Here's how the part is built. I have some questions about the finished solid (model axes, mm). Face numbers are marked on the shaded views. A direction names the side the tool comes from. Round coordinates to 2 decimals unless told otherwise and drop trailing zeros. Order: outer loops, then holes, each group sorted by start corner. A loop starts at its lowest first (then second) coordinate and runs counter-clockwise, first axis right, second up. Notation, with made-up numbers: (51, 46.5) -> (109, 46.5) arc R27 cw to (109, 76.5) -> close; hole circle Ø5 at (87, 38.5). An arc over 180 degrees is marked (long way). Answer in a Markdown table with one row per item.
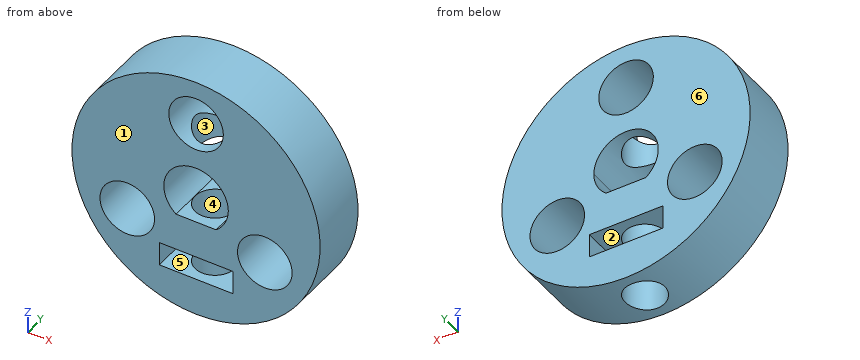
```python
from build123d import *

# Parameters (mm, degrees)
SKETCH1_R                      = 12.5
BOSS_EXTRUDE1_DEPTH            = 6
CUT_EXTRUDE1_REACH             = 20.668
CUT_EXTRUDE2_REACH             = 20.668
SKETCH3_R                      = 2.75
CUT_EXTRUDE3_REACH             = 22.463
SKETCH4_R                      = 2
CUT_EXTRUDE3_DIRECTION_2_REACH = 22.463
CUT_EXTRUDE4_REACH             = 20.668
SKETCH5_W                      = 7.4
SKETCH5_H                      = 2.4


with BuildPart() as part:
    # Sketch1 → Boss-Extrude1 (new body)
    with BuildSketch(Plane(origin=(0, 0, 0), x_dir=(1, 0, 0), z_dir=(0, 1, 0))):
        with Locations(Location((0, 0, 0), (0, 0, 270))):
            Circle(SKETCH1_R)
    extrude(amount=BOSS_EXTRUDE1_DEPTH)

    # Sketch2 → Cut-Extrude1 (cut, up to next)
    with BuildSketch(Plane(origin=(0, 6, 0), x_dir=(1, 0, 0), z_dir=(0, 1, 0)), mode=Mode.PRIVATE) as cut_extrude1_sk1:
        with BuildLine():
            Line((2.014944168, 2.55), (-2.014944168, 2.55))
            ThreePointArc((-2.014944168, 2.55), (-1.416674178, -2.924984491), (3.25, 0))
            ThreePointArc((3.25, 0), (2.924984491, 1.416674178), (2.014944168, 2.55))
        make_face()
    cut_extrude1_tool1 = extrude(cut_extrude1_sk1.sketch, amount=-CUT_EXTRUDE1_REACH, mode=Mode.PRIVATE) & part.part
    add(cut_extrude1_tool1.solids().sort_by_distance((0, 6, 0.174477))[0], mode=Mode.SUBTRACT)

    # Sketch3 → Cut-Extrude2 (cut, up to next)
    with BuildSketch(Plane(origin=(0, 6, 0), x_dir=(1, 0, 0), z_dir=(0, 1, 0)), mode=Mode.PRIVATE) as cut_extrude2_sk1:
        with Locations(Location((0, -8, 0), (0, 0, 270))):
            Circle(SKETCH3_R)
    cut_extrude2_tool1 = extrude(cut_extrude2_sk1.sketch, amount=-CUT_EXTRUDE2_REACH, mode=Mode.PRIVATE) & part.part
    # Sketch3 → Cut-Extrude2 (cut, up to next)
    with BuildSketch(Plane(origin=(0, 6, 0), x_dir=(1, 0, 0), z_dir=(0, 1, 0)), mode=Mode.PRIVATE) as cut_extrude2_sk2:
        with Locations(Location((-6.92820323, 4, 0), (0, 0, 270))):
            Circle(SKETCH3_R)
    cut_extrude2_tool2 = extrude(cut_extrude2_sk2.sketch, amount=-CUT_EXTRUDE2_REACH, mode=Mode.PRIVATE) & part.part
    # Sketch3 → Cut-Extrude2 (cut, up to next)
    with BuildSketch(Plane(origin=(0, 6, 0), x_dir=(1, 0, 0), z_dir=(0, 1, 0)), mode=Mode.PRIVATE) as cut_extrude2_sk3:
        with Locations(Location((6.92820323, 4, 0), (0, 0, 270))):
            Circle(SKETCH3_R)
    cut_extrude2_tool3 = extrude(cut_extrude2_sk3.sketch, amount=-CUT_EXTRUDE2_REACH, mode=Mode.PRIVATE) & part.part
    add(cut_extrude2_tool1.solids().sort_by_distance((0, 6, 8))[0], mode=Mode.SUBTRACT)
    add(cut_extrude2_tool2.solids().sort_by_distance((-6.928203, 6, -4))[0], mode=Mode.SUBTRACT)
    add(cut_extrude2_tool3.solids().sort_by_distance((6.928203, 6, -4))[0], mode=Mode.SUBTRACT)

    # Sketch4 → Cut-Extrude3 (cut, up to next)
    with BuildSketch(Plane.XY.offset(-2.55), mode=Mode.PRIVATE) as cut_extrude3_sk1:
        with Locations(Location((0, 3, 0), (0, 0, 180))):
            Circle(SKETCH4_R)
    cut_extrude3_tool1 = extrude(cut_extrude3_sk1.sketch, amount=-CUT_EXTRUDE3_REACH, mode=Mode.PRIVATE) & part.part
    add(cut_extrude3_tool1.solids().sort_by_distance((0, 3, -2.55))[0], mode=Mode.SUBTRACT)

    # Sketch4 → Cut-Extrude3 direction 2 (cut, up to next)
    with BuildSketch(Plane.XY.offset(-2.55), mode=Mode.PRIVATE) as cut_extrude3_direction_2_sk1:
        with Locations(Location((0, 3, 0), (0, 0, 180))):
            Circle(SKETCH4_R)
    cut_extrude3_direction_2_tool1 = extrude(cut_extrude3_direction_2_sk1.sketch, amount=CUT_EXTRUDE3_DIRECTION_2_REACH, mode=Mode.PRIVATE) & part.part
    add(cut_extrude3_direction_2_tool1.solids().sort_by_distance((0, 3, -2.55))[0], mode=Mode.SUBTRACT)

    # Sketch5 → Cut-Extrude4 (cut, up to next)
    with BuildSketch(Plane(origin=(0, 6, 0), x_dir=(1, 0, 0), z_dir=(0, 1, 0)), mode=Mode.PRIVATE) as cut_extrude4_sk1:
        with Locations((0, 7.525)):
            Rectangle(SKETCH5_W, SKETCH5_H)
    cut_extrude4_tool1 = extrude(cut_extrude4_sk1.sketch, amount=-CUT_EXTRUDE4_REACH, mode=Mode.PRIVATE) & part.part
    add(cut_extrude4_tool1.solids().sort_by_distance((0, 6, -7.525))[0], mode=Mode.SUBTRACT)


solid = part.part
```
1. Suppose I cut it at A-A on z = -4. Write out the boundary of the cut face in (x, y), then the cut area to 3 significant figures.
Numbers:
| item | result |
|---|---|
| outline | (-11.84, 0) -> (-9.68, 0) -> (-9.68, 6) -> (-11.84, 6) -> close; (-4.18, 0) -> (4.18, 0) -> (4.18, 6) -> (-4.18, 6) -> close; (9.68, 0) -> (11.84, 0) -> (11.84, 6) -> (9.68, 6) -> close; hole circle Ø4 at (0, 3) |
| area | 63.5 mm2 |
2. For the marked faces 4, 5 and 6, which set-ups out of +Z, -Z, +X, -X, +Y, -Y let a thin tool reach every point of the face, with its end or its side?
Numbers:
| item | result |
|---|---|
| face 4 | -Z |
| face 5 | +Y, -Y |
| face 6 | +Z, -Z, +X, -X, +Y |
3. Suppose I cut it at C-C on y = 4.25. Write out the boundary of the cut face in (x, z) (3 decimals), then the cut area to 3 significant figures.
Numbers:
| item | result |
|---|---|
| outline | (-3.7, -8.725) -> (-3.7, -6.325) -> (-1.561, -6.325) -> (-1.561, -2.55) -> (-2.015, -2.55) arc R3.25 cw to (-1.561, 2.85) -> (-1.561, 5.736) arc R2.75 cw (long way) to (1.561, 5.736) -> (1.561, 2.85) arc R3.25 cw to (2.015, -2.55) -> (1.561, -2.55) -> (1.561, -6.325) -> (3.7, -6.325) -> (3.7, -8.725) -> (1.561, -8.725) -> (1.561, -12.402) arc R12.5 ccw (long way) to (-1.561, -12.402) -> (-1.561, -8.725) -> close; hole circle Ø5.5 at (-6.928, -4); hole circle Ø5.5 at (6.928, -4) |
| area | 340 mm2 |
4. Suppose I cut it at B-B on x = 0. Write out the boundary of the cut face in (y, z) (3 decimals), then the cut area to 3 significant figures.
Numbers:
| item | result |
|---|---|
| outline | (0, -12.5) -> (1, -12.5) -> (1, -8.725) -> (0, -8.725) -> close; (0, -6.325) -> (1, -6.325) -> (1, -2.55) -> (0, -2.55) -> close; (0, 3.25) -> (1, 3.25) -> (1, 5.25) -> (0, 5.25) -> close; (0, 10.75) -> (6, 10.75) -> (6, 12.5) -> (0, 12.5) -> close; (5, -12.5) -> (6, -12.5) -> (6, -8.725) -> (5, -8.725) -> close; (5, -6.325) -> (6, -6.325) -> (6, -2.55) -> (5, -2.55) -> close; (5, 3.25) -> (6, 3.25) -> (6, 5.25) -> (5, 5.25) -> close |
| area | 29.6 mm2 |
5. Please list where these lines run through material, in increasing order: line 1 along Z through (x, y) = (1, 0.5) (3 decimals); line 2 along X through (y, z) = (1.75, -2.5); line 3 along X through (y, z) = (4.6, -4).
Numbers:
| item | result |
|---|---|
| line 1 | z = -12.46 to -8.725, -6.325 to -2.55, 3.092 to 5.438, 10.562 to 12.46 |
| line 2 | x = -12.25 to -9.23, -4.62 to -2.08, 2.08 to 4.62, 9.23 to 12.25 |
| line 3 | x = -11.84 to -9.68, -4.18 to -1.2, 1.2 to 4.18, 9.68 to 11.84 |
6. Suppose I cut it at D-D on z = 2. Write out the boundary of the cut face in (x, y), then the cut area to 3 significant figures.
Numbers:
| item | result |
|---|---|
| outline | (-12.34, 0) -> (-2.56, 0) -> (-2.56, 6) -> (-12.34, 6) -> close; (2.56, 0) -> (12.34, 0) -> (12.34, 6) -> (2.56, 6) -> close |
| area | 117 mm2 |
7. We'd pull the mould along Y, two halves only. Please class the marked faces 1, 2 and 3: released by +Y, released by -Y, zero draft, split by the parting line, or undercut.
Numbers:
| item | result |
|---|---|
| face 1 | released by -Y |
| face 2 | zero draft |
| face 3 | undercut |
8. For pin 1 Ø2.5 at (y, z) = (3.5, -7.5) entering from +X; pin 2 Ø9 at (x, z) = (0, 8) entering from +Y; pin 3 Ø2 at (y, z) = (2, -7) entering from -X; pin 4 Ø2 at (x, y) = (6, 1.5) entering from -Z, each with a flat end and sliding along its axis, tell me the tip position at first contact or that it passes through.
Numbers:
| item | result |
|---|---|
| pin 1 | stops at x = 10.83 |
| pin 2 | stops at y = 6 |
| pin 3 | stops at x = -10.97 |
| pin 4 | stops at z = -11.46 |
